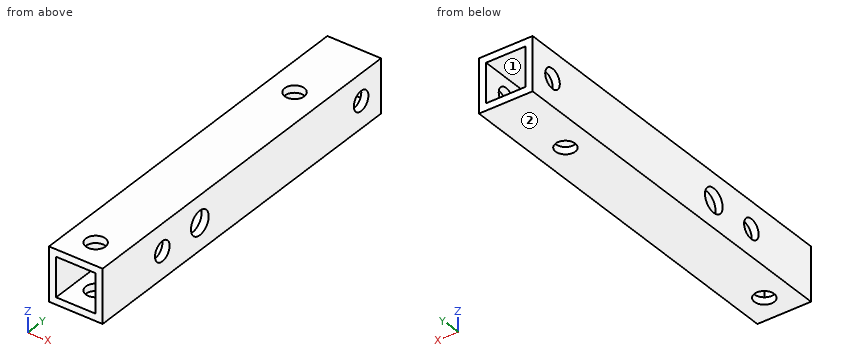
Autodesk Inventor part; units mm, degrees
ref_plane "YZ Plane" through (0, 0, 0) normal (1, 0, 0) x (0, 1, 0)
ref_plane "XZ Plane" through (0, 0, 0) normal (0, 1, 0) x (-1, 0, 0)
ref_plane "XY Plane" through (0, 0, 0) normal (0, 0, 1) x (1, 0, 0)
sketch "スケッチ1" plane through (0, 0, 0) normal (0, 1, 0) x (-1, 0, 0)
  line L0 (0, 0) -> (-9, 0)
  line L1 (-9, 0) -> (-9, 9)
  line L2 (-9, 9) -> (0, 9)
  line L3 (0, 9) -> (0, 0)
  line L4 (-1.2, 7.8) -> (-7.8, 7.8)
  line L5 (-7.8, 7.8) -> (-7.8, 1.2)
  line L6 (-7.8, 1.2) -> (-1.2, 1.2)
  line L7 (-1.2, 1.2) -> (-1.2, 7.8)
  dimension "d0" = 9
  dimension "d1" = 9
  dimension "d2" = 1.2
  dimension "d3" = 1.2
  dimension "d4" = 1.2
  dimension "d5" = 1.2
extrude "押し出し1" add sketch "スケッチ1" along normal blind 120.5
sketch "スケッチ3" plane through (9, 0, 9) normal (1, 0, 0) x (0, 0, -1)
  line L0 (0, 120.5) -> (9, 120.5)
  line L1 (9, 0) -> (9, 120.5)
  line L2 (0, 0) -> (9, 0)
  point P0 (4.5, 71)
  point P1 (4.5, 116)
  dimension "d20" = 4.5
  dimension "d38" = 71
  dimension "d39" = 45
hole "穴2" at (9, 71, 4.5) at (9, 116, 4.5) direction (-1, 0, 0) diameter 3.3 end through all
sketch "スケッチ4" plane through (0, 0, 9) normal (0, 0, 1) x (1, 0, 0)
  line L0 (0, 120.5) -> (9, 120.5)
  line L1 (9, 0) -> (9, 120.5)
  line L2 (0, 0) -> (9, 0)
  point P0 (4.5, 62)
  point P1 (4.5, 107)
  dimension "d29" = 4.5
  dimension "d37" = 62
  dimension "d40" = 45
hole "穴3" at (4.5, 62, 9) at (4.5, 107, 9) direction (0, 0, -1) diameter 3.3 end through all
sketch "スケッチ5" plane through (9, 0, 9) normal (1, 0, 0) x (0, 0, -1)
  line L0 (0, 0) -> (0, 120.5)
  circle A0 centre (4.5, 71) radius 1.65
  point P0 (9, 0)
  point P1 (4.5, 79.5)
  dimension "d41" = 4.5
  dimension "d42" = 8.5
hole "穴4" at (9, 79.5, 4.5) direction (-1, 0, 0) diameter 4 end through all
sketch "スケッチ6" plane through (0, 0, 0) normal (0, -1, 0) x (1, 0, 0)
  line L0 (9, 0) -> (0, 0)
  line L1 (0, 9) -> (9, 9)
  line L2 (0, 0) -> (9, 0)
  line L3 (9, 0) -> (9, 9)
  line L4 (9, 9) -> (0, 9)
  line L5 (0, 9) -> (0, 0)
  line L6 (1.2, 1.2) -> (7.8, 1.2)
  line L7 (7.8, 1.2) -> (7.8, 7.8)
  line L8 (1.2, 1.2) -> (7.8, 1.2)
  line L9 (7.8, 1.2) -> (7.8, 7.8)
  line L10 (7.8, 7.8) -> (1.2, 7.8)
  line L11 (1.2, 7.8) -> (1.2, 1.2)
extrude "押し出し2" cut sketch "スケッチ6" against normal blind 57.5
equation "\"d3\" = d2"
equation "\"d4\" = d2"
equation "\"d5\" = d3"
properties part number "ハンド9x9_1" material "アルミニウム 6061"
The model under review builds one solid part; all positions refer to its coordinate system, in mm. Face numbers are marked on the shaded views. A direction names the side the tool comes from. Coordinates: 2 decimals unless noted, no trailing zeros. Order: outer loops, then holes, each group sorted by start corner. A loop starts at its lowest first (then second) coordinate and runs counter-clockwise, first axis right, second up. Notation, with made-up numbers: (-19, 17.25) -> (29, 17.25) arc R18 ccw to (29, 25.25) -> close; hole circle Ø9 at (-35, 72.25). An arc over 180 degrees is marked (long way). Answer in a Markdown table with one row per item. Add a question column.
Item 1: Clearance check with a flat-ended pin moving along its axis: pin 1 (5 mm diameter, centred on y = 79.5, z = 4.5, fed in from +X). State where the tip first meets the part, or that it passes through.
Item 2: We need section A-A on z = 4.5. Give the number of separate pieces and of enclosed holes in the cut face, plus the area to 3 significant figures.
Item 3: We need section C-C on y = 67. Write out the cut boundary in (x, z).
Item 4: We need section D-D on y = 116. Write out the cut boundary in (x, z), plus the area to 3 significant figures.
Item 5: Machinability: for the marked faces 1 and 2, which of the approach directions +Z, -Z, +X, -X, +Y, -Y give a long, thin tool a straight path to every point of the face, cutting with its end or side? Answer none if there is none.
Item 6: To check wall thickness, follow probe 1 along Y at (x, z) = (0.8, 4.5); probe 2 along Y at (x, z) = (4.5, 0.65); probe 3 along Z at (x, y) = (3, 117). State the ranges of each line that lie inside material, in increasing order.
Item 7: We need section B-B on y = 79.5. Write out the cut boundary in (x, z).
Final values:
| question | item | result |
|---|---|---|
| 1 | pin 1 | stops at x = 9 |
| 2 | separate pieces | 8 |
| 2 | enclosed holes | 0 |
| 2 | area | 126 mm2 |
| 3 | outline | (0, 0) -> (9, 0) -> (9, 9) -> (0, 9) -> close; hole (1.2, 1.2) -> (7.8, 1.2) -> (7.8, 7.8) -> (1.2, 7.8) -> close |
| 4 | outline | (0, 0) -> (9, 0) -> (9, 2.85) -> (7.8, 2.85) -> (7.8, 1.2) -> (1.2, 1.2) -> (1.2, 2.85) -> (0, 2.85) -> close; (0, 6.15) -> (1.2, 6.15) -> (1.2, 7.8) -> (7.8, 7.8) -> (7.8, 6.15) -> (9, 6.15) -> (9, 9) -> (0, 9) -> close |
| 4 | area | 29.5 mm2 |
| 5 | face 1 | +Y, -Y |
| 5 | face 2 | -Z, +X, -X, +Y, -Y |
| 6 | probe 1 | y = 57.5 to 69.35, 72.65 to 77.5, 81.5 to 114.35, 117.65 to 120.5 |
| 6 | probe 2 | y = 57.5 to 60.35, 63.65 to 105.35, 108.65 to 120.5 |
| 6 | probe 3 | z = 0 to 1.2, 7.8 to 9 |
| 7 | outline | (0, 0) -> (9, 0) -> (9, 2.5) -> (7.8, 2.5) -> (7.8, 1.2) -> (1.2, 1.2) -> (1.2, 2.5) -> (0, 2.5) -> close; (0, 6.5) -> (1.2, 6.5) -> (1.2, 7.8) -> (7.8, 7.8) -> (7.8, 6.5) -> (9, 6.5) -> (9, 9) -> (0, 9) -> close |
